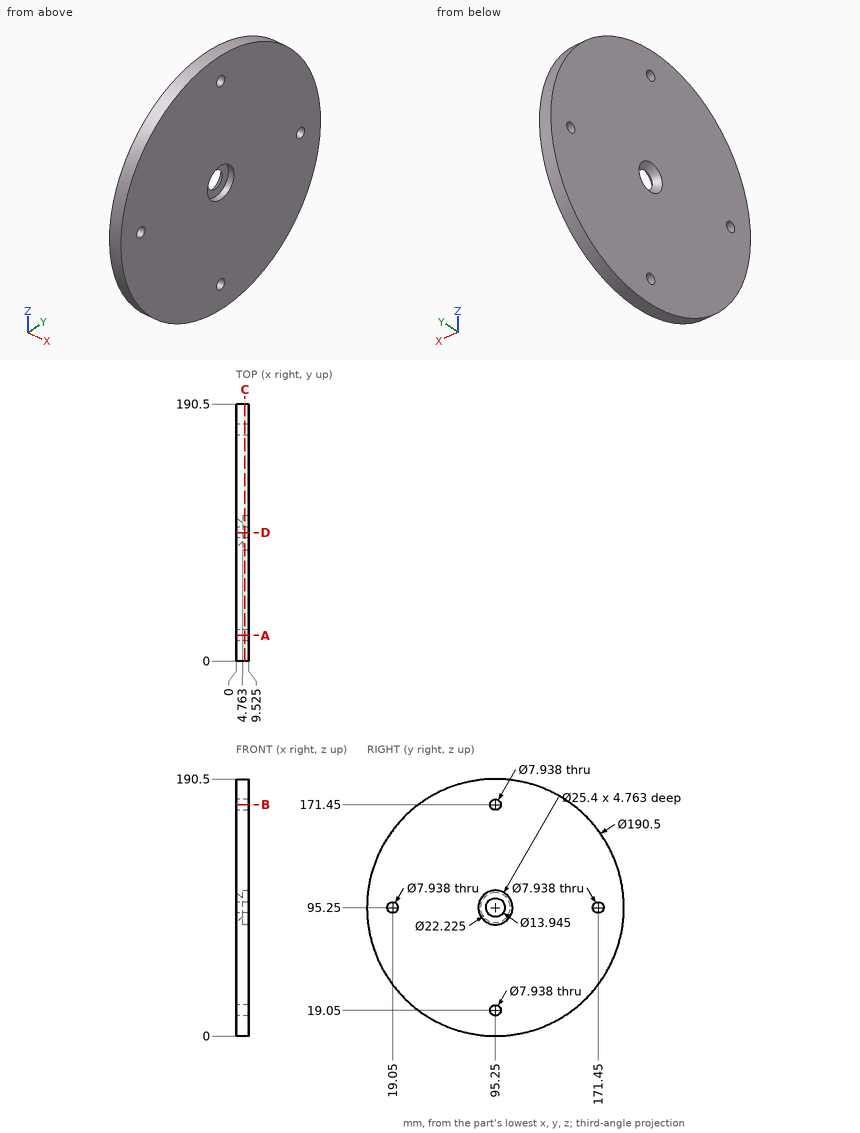
Drawing for the job (mm, zero at the part's lowest x, y, z). Coordinates: 2 decimals unless noted, no trailing zeros. Write each loop counter-clockwise with the first axis right and the second up, starting at its lowest first coordinate (ties: lowest second). Pieces come first, ordered by that corner, then holes. Notation, with made-up numbers: (-6.75, 59.25) -> (42.25, 59.25) arc R13 cw to (42.25, 84.25) -> close; hole circle Ø11 at (69.25, 81). An arc over 180 degrees is marked (long way). One line per item, written item: value. Start each with the question number.
1) Slice it at C-C on x = 6.5. Write the cut outline in (y, z).
2) Flat gauge pins, fed straight in: pin 1 Ø1 at (x, y) = (4.5, 149.5) entering from -Z (1 decimal); pin 2 Ø2 at (x, y) = (4.5, 50.5) entering from +Z; pin 3 Ø2 at (x, z) = (5, 98) entering from +Y; pin 4 Ø5 at (y, z) = (19.05, 95.25) entering from +X. Where does each tip first touch, or does it go through?
3) Probe probe 1 along Y at (x, z) = (6.5, 95.25); probe 2 along Y at (x, z) = (3, 95.25) (1 decimal); probe 3 along Z at (x, y) = (7.75, 171.45). List the from-to ranges inside material, lowest first.
4) Slice it at A-A on y = 19.05. Write the cut outline in (x, z) (1 decimal).
5) Slice it at D-D on y = 95.25. Count the separate pieces of the cut face and the enclosed holes in it, then the cut area to 3 significant figures.
Answers follow:
1. outline: circle Ø190.5 at (95.25, 95.25); hole circle Ø7.94 at (19.05, 95.25); hole circle Ø25.4 at (95.25, 95.25); hole circle Ø7.94 at (95.25, 19.05); hole circle Ø7.94 at (95.25, 171.45); hole circle Ø7.94 at (171.45, 95.25)
2. pin 1: z = 16.6
2. pin 2: z = 179.86
2. pin 3: y = 190.48
2. pin 4: through
3. probe 1: 0 to 15.08, 23.02 to 82.55, 107.95 to 167.48, 175.42 to 190.5
3. probe 2: 0 to 15.1, 23 to 86.7, 103.8 to 167.5, 175.4 to 190.5
3. probe 3: 38.1 to 91.28, 99.22 to 152.4
4. outline: (0, 38.1) -> (9.5, 38.1) -> (9.5, 91.3) -> (0, 91.3) -> close; (0, 99.2) -> (9.5, 99.2) -> (9.5, 152.4) -> (0, 152.4) -> close
5. separate pieces: 4
5. enclosed holes: 0
5. area: 1,460 mm2
